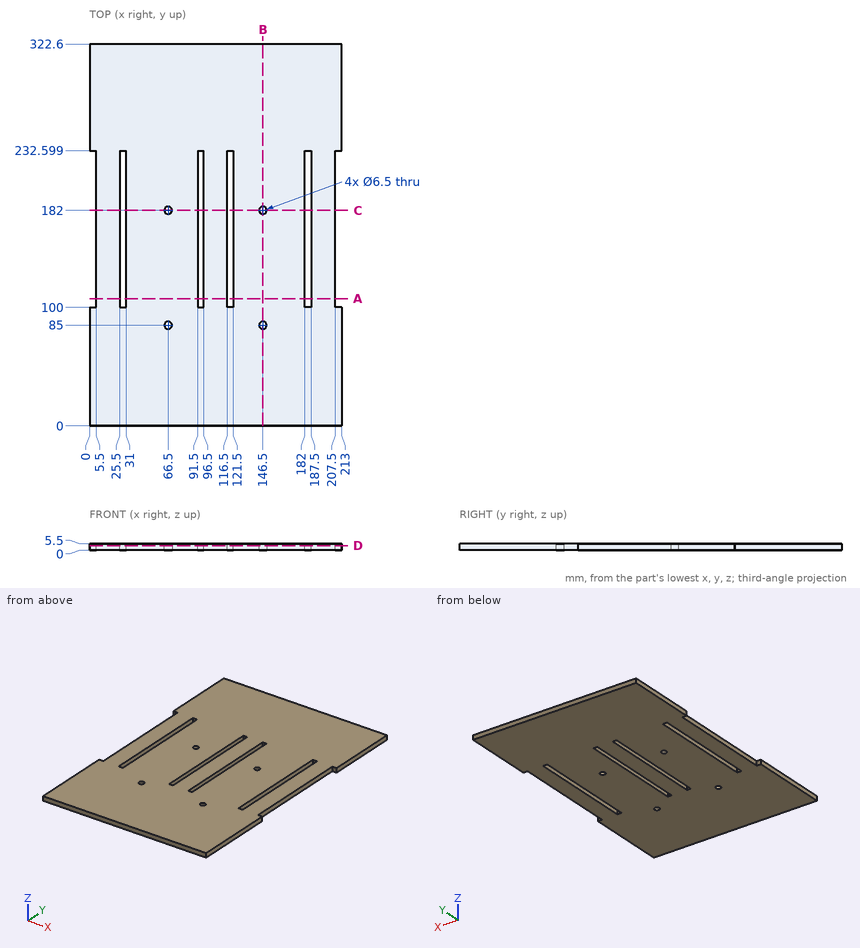
Geometry check sheet. Reference: drawing and pictorial views, mm from the part's lowest x, y, z. Coordinates: 2 decimals unless noted, no trailing zeros. Write each loop counter-clockwise with the first axis right and the second up, starting at its lowest first coordinate (ties: lowest second). Pieces come first, ordered by that corner, then holes.
Item 1: Scan lines: probe 1 along Y at (x, z) = (66.5, 4.4); probe 2 along X at (y, z) = (231, 2.8); probe 3 along Y at (x, z) = (26.5, 1). Record each from-to range of solid material in increasing order.
Numbers:
probe 1: y = 0 to 81.75, 88.25 to 178.75, 185.25 to 322.6
probe 2: x = 5.5 to 25.5, 31 to 91.5, 96.5 to 116.5, 121.5 to 182, 187.5 to 207.5
probe 3: y = 0 to 100, 232.6 to 322.6
Item 2: Cross-section at B-B on x = 146.5. Record the boundary of the cut face in (y, z), then the cut area to 3 significant figures.
Numbers:
outline: (0, 0) - (81.75, 0) - (81.75, 5.5) - (0, 5.5) - close; (88.25, 0) - (178.75, 0) - (178.75, 5.5) - (88.25, 5.5) - close; (185.25, 0) - (322.6, 0) - (322.6, 5.5) - (185.25, 5.5) - close
area: 1,700 mm2
Item 3: Depth check by flat-ended pin: pin 1 Ø5 at (x, y) = (146.5, 85) entering from +Z; pin 2 Ø1.5 at (y, z) = (63.5, 0.5) entering from -X; pin 3 Ø1.6 at (y, z) = (169.5, 2.5) entering from +X; pin 4 Ø3 at (y, z) = (134.5, 2) entering from -X. Enter the tip coordinate at first touch or a pass-through.
Numbers:
pin 1: passes through
pin 2: stops at x = 0
pin 3: stops at x = 207.5
pin 4: stops at x = 5.5
Item 4: Cross-section at D-D on z = 4.1. Count the separate pieces of the cut face and the enclosed holes in it, then the cut area to 3 significant figures.
Numbers:
separate pieces: 1
enclosed holes: 8
area: 64,300 mm2
Item 5: Cross-section at C-C on y = 182. Record the boundary of the cut face in (x, z).
Numbers:
outline: (5.5, 0) - (25.5, 0) - (25.5, 5.5) - (5.5, 5.5) - close; (31, 0) - (63.25, 0) - (63.25, 5.5) - (31, 5.5) - close; (69.75, 0) - (91.5, 0) - (91.5, 5.5) - (69.75, 5.5) - close; (96.5, 0) - (116.5, 0) - (116.5, 5.5) - (96.5, 5.5) - close; (121.5, 0) - (143.25, 0) - (143.25, 5.5) - (121.5, 5.5) - close; (149.75, 0) - (182, 0) - (182, 5.5) - (149.75, 5.5) - close; (187.5, 0) - (207.5, 0) - (207.5, 5.5) - (187.5, 5.5) - close
Item 6: Cross-section at A-A on y = 107.5. Record the boundary of the cut face in (x, z), then the cut area to 4 significant figures.
Numbers:
outline: (5.5, 0) - (25.5, 0) - (25.5, 5.5) - (5.5, 5.5) - close; (31, 0) - (91.5, 0) - (91.5, 5.5) - (31, 5.5) - close; (96.5, 0) - (116.5, 0) - (116.5, 5.5) - (96.5, 5.5) - close; (121.5, 0) - (182, 0) - (182, 5.5) - (121.5, 5.5) - close; (187.5, 0) - (207.5, 0) - (207.5, 5.5) - (187.5, 5.5) - close
area: 995.5 mm2
